For this review, take the finished solid that the model builds, in its own axes (mm). Face numbers are marked on the shaded views. A direction names the side the tool comes from. Coordinates: 2 decimals unless noted, no trailing zeros. Order: outer loops, then holes, each group sorted by start corner. A loop starts at its lowest first (then second) coordinate and runs counter-clockwise, first axis right, second up. Notation, with made-up numbers: (61.5, -14) -> (77.5, -14) arc R26 ccw to (77.5, 6) -> close; hole circle Ø10 at (-1.75, 48.5). An arc over 180 degrees is marked (long way). Answer as a JSON object with one key per item and string values. Group by question number.
1) Add section A-A, the plane y = -18. Write out the cut boundary in (x, z).
2) Add section C-C, the plane z = 5.25. Write out the cut boundary in (x, y), then the cut area to 3 significant figures.
3) Draft analysis for pull direction Y (two halves, no side actions). For the marked faces 3, 4, 5 and 6, state which applies: +Y half, -Y half, draft (parallel to the pull), parting line (faces both ways), or undercut.
4) For pin 1 (5 mm diameter, centred on x = 33.5, y = -1.5, fed in from +Z); pin 2 (4 mm diameter, centred on x = 10.5, y = -14, fed in from -Z); pin 3 (3 mm diameter, centred on y = -44, z = 3, fed in from +X); pin 4 (3.5 mm diameter, centred on x = 58.5, z = 10, fed in from -Y), all flat-tipped, find the tip position at first contact; note any pin that passes through.
5) Wall thickness on L1, parallel to X at y = -19, z = 2.25; L2, parallel to X at y = -36, z = 11.5; L3, parallel to Z at x = 39.5, y = -10: over which ranges is each line inside the solid? List them lowest first.
6) Machinability: for the marked faces 1 and 2, which of the approach directions +Z, -Z, +X, -X, +Y, -Y give a long, thin tool a straight path to every point of the face, cutting with its end or side? Answer none if there is none.
7) Add section D-D, the plane y = 11. Write out the cut boundary in (x, z).
8) Add section B-B, the plane x = -10. Write out the cut boundary in (y, z).
from build123d import *

# Parameters (mm, degrees)
F0_W     = 12
F0_H     = 50
F1_DEPTH = 4
F2_W     = 103
F2_H     = 59
F3_DEPTH = 8
F4_DEPTH = 15
F5_DEPTH = 2


with BuildPart() as f1:
    # F0 (on Top) → F1 (new body)
    with BuildSketch(Plane.XY):
        Polygon((-39.061178, 17.013159), (-57.475254, 17.013159), (-57.475254, -47.986841), (52.524746, -47.986841), (52.524746, -40.486841), (52.524746, 9.513159), (52.524746, 17.013159), (10.938822, 17.013159), align=None)
        with Locations((58.524746, -15.486841)):
            Rectangle(F0_W, F0_H)
    extrude(amount=F1_DEPTH)

    # F2 (on face) → F3 (cut)
    with BuildSketch(Plane.XY.offset(4)):
        with Locations((-2.536587, -14.736841)):
            Rectangle(F2_W, F2_H)
    extrude(amount=-F3_DEPTH, mode=Mode.SUBTRACT)

    # F0 (on Top) → F4 (join)
    with BuildSketch(Plane.XY):
        with Locations((58.524746, -15.486841)):
            Rectangle(F0_W, F0_H)
    extrude(amount=F4_DEPTH)

    # F0 (on Top) → F5 (join)
    with BuildSketch(Plane.XY):
        Polygon((-39.061178, 17.013159), (-57.475254, 17.013159), (-57.475254, -47.986841), (52.524746, -47.986841), (52.524746, -40.486841), (52.524746, 9.513159), (52.524746, 17.013159), (10.938822, 17.013159), align=None)
    extrude(amount=F5_DEPTH)


solid = f1.part
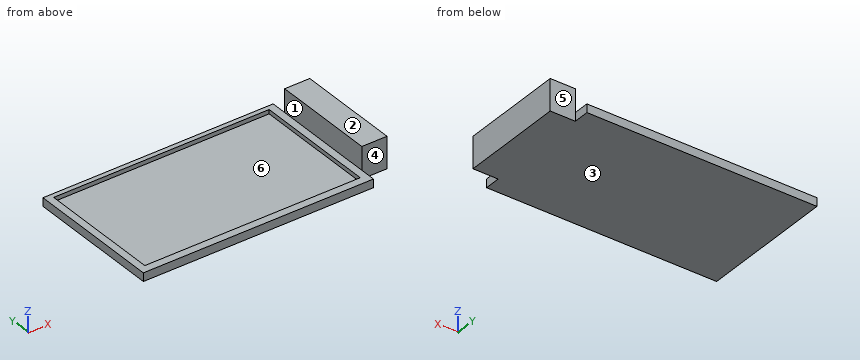
Output values:
{
 "1": {"outline": "(-57.48, 0) -> (64.52, 0) -> (64.52, 15) -> (52.52, 15) -> (52.52, 4) -> (48.96, 4) -> (48.96, 2) -> (-54.04, 2) -> (-54.04, 4) -> (-57.48, 4) -> close"},
 "2": {"outline": "(52.52, -40.49) -> (64.52, -40.49) -> (64.52, 9.51) -> (52.52, 9.51) -> close", "area": "600 mm²"},
 "3": {"face 3": "draft", "face 4": "-Y half", "face 5": "+Y half", "face 6": "undercut"},
 "4": {"pin 1": "stops at z = 2", "pin 2": "stops at z = 0", "pin 3": "stops at x = 52.52", "pin 4": "stops at y = -40.49"},
 "5": {"L1": "x = -57.48 to -54.04, 48.96 to 64.52", "L2": "x = 52.52 to 64.52", "L3": "z = 0 to 2"},
 "6": {"face 1": "+Z, -X, +Y, -Y", "face 2": "+Z, +X, -X, +Y, -Y"},
 "7": {"outline": "(-57.48, 0) -> (52.52, 0) -> (52.52, 4) -> (48.96, 4) -> (48.96, 2) -> (-54.04, 2) -> (-54.04, 4) -> (-57.48, 4) -> close"},
 "8": {"outline": "(-47.99, 0) -> (17.01, 0) -> (17.01, 4) -> (14.76, 4) -> (14.76, 2) -> (-44.24, 2) -> (-44.24, 4) -> (-47.99, 4) -> close"}
}
